Design review of the part built by this model. Coordinates are the model's own, in mm. A direction names the side the tool comes from. Give positions to 0.01 mm unless a question says otherwise; leave off trailing zeros. Loops run counter-clockwise (first coordinate to the right, second up) from the corner with the lowest first, then second, coordinate; pieces in that order, holes last.
from build123d import *

# Parameters (mm, degrees)
SKETCH1_W                    = 152.4
SKETCH1_H                    = 114.3
BOSS_EXTRUDE1_DEPTH          = 38.1
SKETCH2_W                    = 457.2
SKETCH2_H                    = 38.1
BOSS_EXTRUDE2_DEPTH          = 19.05
F_96_0_0063_DIAMETER_HOLE1_D = 19.05


with BuildPart() as part:
    # Sketch1 → Boss-Extrude1 (new body)
    with BuildSketch(Plane(origin=(0, 0, 0), x_dir=(1, 0, 0), z_dir=(0, 1, 0))):
        with Locations((76.2, 57.15)):
            Rectangle(SKETCH1_W, SKETCH1_H)
    extrude(amount=BOSS_EXTRUDE1_DEPTH)

    # Sketch2 → Boss-Extrude2 (add)
    with BuildSketch(Plane(origin=(0, 0, -114.3), x_dir=(-1, 0, 0), z_dir=(0, 0, -1))):
        with Locations((-76.2, 19.05)):
            Rectangle(SKETCH2_W, SKETCH2_H)
    extrude(amount=BOSS_EXTRUDE2_DEPTH)

    # #96 (0.0063) Diameter Hole1 (through all)
    with Locations(Plane(origin=(76.2, 0, -22.86), x_dir=(0, 0, -1), z_dir=(0, -1, 0))):
        with Locations((0, 0)):
            Hole(F_96_0_0063_DIAMETER_HOLE1_D / 2)


solid = part.part
Q1. Wall thickness on line 1 (Z direction, x = 76, y = 23); line 2 (X direction, y = 23.5, z = -22.86) (3 decimals); line 3 (X direction, y = 33.5, z = -106): over which ranges is each line inside the solid? List them lowest first.
Results:
line 1: z = -133.35 to -32.38, -13.34 to 0
line 2: x = 0 to 66.675, 85.725 to 152.4
line 3: x = 0 to 152.4
Q2. Tool access review of faces 1 (the face through (152.4, 19, -56)), 2 (the face through (75, 19, 0)), 3 (the face through (0, 19, -56)): name each direction out of +Z, -Z, +X, -X, +Y, -Y from which nothing blocks a thin tool from reaching the whole face with its end or side.
Results:
face 1: +Z, +X, +Y, -Y
face 2: +Z, +X, -X, +Y, -Y
face 3: +Z, -X, +Y, -Y
Q3. Take a section at B-B (x = 76.2). Give the boundary of the cut face in (y, z) (3 decimals).
Results:
outline: (0, -133.35) - (38.1, -133.35) - (38.1, -32.385) - (0, -32.385) - close; (0, -13.335) - (38.1, -13.335) - (38.1, 0) - (0, 0) - close
Q4. Draft analysis for pull direction Z (two halves, no side actions). For faces 4 (the face through (304.8, 19, -124)), 5 (the face through (-75, 19, -114.3)), 6 (the face through (70.404, 19.317, -30.419)), state which applies: pulls with the +Z half, pulls with the -Z half, needs draft (parallel to the pull), parting line crosses it, or undercut.
Results:
face 4: needs draft
face 5: pulls with the +Z half
face 6: undercut
Q5. Insertion check: pin 1 (19 mm diameter, centred on x = 205, y = 20.5, fed in from +Z); pin 2 (19 mm diameter, centred on y = 26.5, z = -54.5, fed in from -X); pin 3 (1.5 mm diameter, centred on y = 34, z = -108, fed in from +X); pin 4 (11.5 mm diameter, centred on x = 76.2, z = -22.86, fed in from +Y). Each pin has a flat end and moves straight along its axis. Give the tip position at first contact, or say it passes through.
Results:
pin 1: stops at z = -114.3
pin 2: stops at x = 0
pin 3: stops at x = 152.4
pin 4: passes through
Q6. Take a section at C-C (y = 24). Give the boundary of the cut face in (x, z) (3 decimals).
Results:
outline: (-152.4, -133.35) - (304.8, -133.35) - (304.8, -114.3) - (152.4, -114.3) - (152.4, 0) - (0, 0) - (0, -114.3) - (-152.4, -114.3) - close; hole circle Ø19.05 at (76.2, -22.86)
Q7. Take a section at A-A (z = -22.86). Give the boundary of the cut face in (x, y) (3 decimals).
Results:
outline: (0, 0) - (66.675, 0) - (66.675, 38.1) - (0, 38.1) - close; (85.725, 0) - (152.4, 0) - (152.4, 38.1) - (85.725, 38.1) - close
Q8. Take a section at D-D (z = -104.5). Give the boundary of the cut face in (x, y).
Results:
outline: (0, 0) - (152.4, 0) - (152.4, 38.1) - (0, 38.1) - close
